Work out the finished part from the listing and answer in its coordinate system (mm). A direction names the side the tool comes from. Round coordinates to 2 decimals unless told otherwise and drop trailing zeros. Use CSV: the item, a comma, the result in double quotes.
from build123d import *

# Parameters (mm, degrees)
F0_R      = 50
F1_DEPTH  = 30
F2_R      = 10
F3_R      = 43
F4_DEPTH  = 27
F6_W      = 12.5
F6_H      = 30
F7_DEPTH  = 9
F9_R      = 45
F10_DEPTH = 3.85
F12_R     = 1.5
F13_DEPTH = 4
F14_DEPTH = 29
F18_DEPTH = 9


with BuildPart() as f1:
    # F0 (on Top) → F1 (new body)
    with BuildSketch(Plane.XY):
        Circle(F0_R)
    extrude(amount=F1_DEPTH)

    # F2
    f2_edges = [f1.edges().sort_by_distance(p)[0] for p in [
        (-50, 0, 30),
        (-50, 0, 0),
    ]]
    fillet(f2_edges, radius=F2_R)

    # F3 (on face) → F4 (cut)
    with BuildSketch(Plane.XY.offset(30)):
        Circle(F3_R)
    extrude(amount=-F4_DEPTH, mode=Mode.SUBTRACT)

    # F6 (on offset) → F7 (cut)
    with BuildSketch(Plane.XZ.offset(50)):
        with Locations((-6.25, 15)):
            Rectangle(F6_W, F6_H)
        with Locations((6.25, 15)):
            Rectangle(F6_W, F6_H)
    extrude(amount=-F7_DEPTH, mode=Mode.SUBTRACT)

    # F9 (on offset) → F10 (cut)
    with BuildSketch(Plane.XY.offset(30)):
        Circle(F9_R)
    extrude(amount=-F10_DEPTH, mode=Mode.SUBTRACT)

    # F12 (on offset) → F13 (cut)
    with BuildSketch(Plane.YZ.offset(-12.5)):
        with Locations((-41.1430431543, 3)):
            Circle(F12_R)
    extrude(amount=-F13_DEPTH, mode=Mode.SUBTRACT)

    # F12 (on offset) → F14 (cut)
    with BuildSketch(Plane.YZ.offset(-12.5)):
        with Locations((-41.1430431543, 3)):
            Circle(F12_R)
    extrude(amount=F14_DEPTH, mode=Mode.SUBTRACT)

    # F15 (on offset) → F17 (revolve)
    with BuildSketch(Plane.YZ.offset(-12.5)):
        with BuildLine():
            Line((-43.2290411645, 28.6602540378), (-43.2290411645, 27.1602540378))
            ThreePointArc((-43.2290411645, 27.1602540378), (-42.9790411645, 27.9102540378), (-43.2290411645, 28.6602540378))
        make_face()
    revolve(axis=Axis((0, 0, 24.574), (0, 0, 1)))

    # F6 (on offset) → F18 (cut)
    with BuildSketch(Plane.XZ.offset(50)):
        with Locations((-6.25, 15)):
            Rectangle(F6_W, F6_H)
        with Locations((6.25, 15)):
            Rectangle(F6_W, F6_H)
    extrude(amount=-F18_DEPTH, mode=Mode.SUBTRACT)


solid = f1.part
(1) For faces 1 (the flat face through (-16.5, -41, 3)), 2 (the flat face through (-1, 2, 3)), 3 (the flat face through (-12.5, -45, 14)), determine the directions among +Z, -Z, +X, -X, +Y, -Y from which every point of the face is accessible in a straight line to the end or side of a thin tool.
Findings below:
face 1,"none"
face 2,"+Z"
face 3,"+Z, -Z, -Y"
(2) The mould has two halves that part along Y. Classify faces 4 (the cylindrical face through (2.02, 49.96, 14.93)), 5 (the flat face through (-1, 1, 0)), 6 (the flat face through (16.5, -41, 3)): released by +Y, released by -Y, zero draft, split by the parting line, or undercut.
Findings below:
face 4,"split by the parting line"
face 5,"zero draft"
face 6,"undercut"
(3) Find the intervals of material crossed by L1, parallel to X at y = 0, z = 12; L2, parallel to Z at x = -4.5, y = -24.5; L3, parallel to X at y = -8.5, z = 23.5, in increasing order. Write a range as from..to.
Findings below:
L1,"x = -50..-43, 43..50"
L2,"z = 0..3"
L3,"x = -48.63..-42.15, 42.15..48.63"
(4) Each of these flat-tipped pins is pushed along its axis until it touches: pin 1 (3 mm diameter, centred on x = -37, z = 15.5, fed in from +Y); pin 2 (12 mm diameter, centred on x = -14, z = 15, fed in from +Y); pin 3 (10 mm diameter, centred on x = -23, z = 9, fed in from +Y); pin 4 (1.5 mm diameter, centred on y = -0.5, z = 20, fed in from +X). Where does it stop, or does it pass through?
Findings below:
pin 1,"stops at y = 35.21"
pin 2,"stops at y = 49.36"
pin 3,"stops at y = 46.63"
pin 4,"stops at x = 50"
